The model under review builds one solid part; all positions refer to its coordinate system, in mm. A direction names the side the tool comes from. Coordinates: 2 decimals unless noted, no trailing zeros. Order: outer loops, then holes, each group sorted by start corner. A loop starts at its lowest first (then second) coordinate and runs counter-clockwise, first axis right, second up.
Autodesk Inventor part; units mm, degrees
ref_plane "YZ Plane" through (0, 0, 0) normal (1, 0, 0) x (0, 1, 0)
ref_plane "XZ Plane" through (0, 0, 0) normal (0, 1, 0) x (-1, 0, 0)
ref_plane "XY Plane" through (0, 0, 0) normal (0, 0, 1) x (1, 0, 0)
sketch "Sketch1" plane through (0, 0, 0) normal (0, 1, 0) x (-1, 0, 0)
  line L0 (0, 0) -> (-155, 0)
  line L1 (-155, 0) -> (-155, -65)
  line L2 (-155, -65) -> (0, -65)
  line L3 (0, -65) -> (0, 0)
  dimension "d0" = 155
  dimension "d1" = 65
extrude "Extrusion1" add sketch "Sketch1" along normal blind 4
sketch "Sketch2" plane through (0, 0, 0) normal (0, -1, 0) x (1, 0, 0)
  line L0 (155, 0) -> (155, -65)
  line L1 (0, 0) -> (155, 0)
  line L2 (0, -65) -> (0, 0)
  line L3 (155, -65) -> (0, -65)
  line L4 (3, -62) -> (3, -3)
  line L5 (3, -3) -> (152, -3)
  line L6 (152, -3) -> (152, -62)
  line L7 (152, -62) -> (3, -62)
  line L8 (152, -62) -> (143, -62)
  line L9 (143, -62) -> (143, -53)
  line L10 (143, -53) -> (152, -53)
  line L11 (152, -53) -> (152, -62)
  circle A0 centre (147.5, -57.5) radius 1.6
  dimension "d4" = 3
  dimension "d5" = 9
  dimension "d6" = 9
  dimension "d7" = 3.2
extrude "Extrusion2" cut sketch "Sketch2" against normal blind 4 contours A0
sketch "Sketch3" plane through (0, 4, 0) normal (0, 1, 0) x (1, 0, 0)
  circle A0 centre (147.5, 57.5) radius 1.6
  line L0 (155, 0) -> (155, 65)
  line L1 (155, 65) -> (0, 65)
  line L2 (0, 65) -> (0, 0)
  line L3 (0, 0) -> (155, 0)
  circle A1 centre (147.5, 57.5) radius 3
  dimension "d10" = 6
extrude "Extrusion3" cut sketch "Sketch3" against normal blind 1 contours A1
sketch "Sketch4" plane through (0, 0, 0) normal (0, -1, 0) x (1, 0, 0)
  circle A0 centre (147.5, -57.5) radius 1.6
  line L0 (155, 0) -> (155, -65)
  line L1 (0, 0) -> (155, 0)
  line L2 (0, -65) -> (0, 0)
  line L3 (155, -65) -> (0, -65)
  line L4 (3, -62) -> (3, -3)
  line L5 (3, -3) -> (152, -3)
  line L6 (152, -3) -> (152, -62)
  line L7 (152, -62) -> (3, -62)
  line L8 (152, -3) -> (143, -3)
  line L9 (143, -3) -> (143, -12)
  line L10 (143, -12) -> (152, -12)
  line L11 (152, -12) -> (152, -3)
  line L12 (3, -3) -> (12, -3)
  line L13 (12, -3) -> (12, -12)
  line L14 (12, -12) -> (3, -12)
  line L15 (3, -12) -> (3, -3)
  line L16 (3, -62) -> (12, -62)
  line L17 (12, -62) -> (12, -53)
  line L18 (12, -53) -> (3, -53)
  line L19 (3, -53) -> (3, -62)
  circle A1 centre (147.5, -7.5) radius 1.6
  circle A2 centre (7.5, -7.5) radius 1.6
  circle A3 centre (7.5, -57.5) radius 1.6
  dimension "d13" = 3
  dimension "d14" = 9
  dimension "d15" = 9
  dimension "d16" = 9
  dimension "d17" = 9
  dimension "d18" = 9
  dimension "d19" = 9
  dimension "d20" = 3.2
  dimension "d21" = 3.2
  dimension "d22" = 3.2
extrude "Extrusion4" cut sketch "Sketch4" against normal blind 4 contours A1 | A2 | A3
sketch "Sketch5" plane through (0, 4, 0) normal (0, 1, 0) x (1, 0, 0)
  circle A0 centre (7.5, 57.5) radius 1.6
  circle A1 centre (7.5, 7.5) radius 1.6
  circle A2 centre (147.5, 7.5) radius 1.6
  circle A3 centre (147.5, 57.5) radius 3
  line L0 (155, 0) -> (155, 65)
  line L1 (155, 65) -> (0, 65)
  line L2 (0, 65) -> (0, 0)
  line L3 (0, 0) -> (155, 0)
  circle A4 centre (7.5, 57.5) radius 3
  circle A5 centre (7.5, 7.5) radius 3
  circle A6 centre (147.5, 7.5) radius 3
  dimension "d25" = 6
  dimension "d26" = 6
  dimension "d27" = 6
extrude "Extrusion5" cut sketch "Sketch5" against normal blind 1 contours A4 | A5 | A6
fillet "Fillet1" radius 3 4 edges at (0, 2, 0) (0, 2, -65) (155, 2, 0) (155, 2, -65)
sketch "Sketch6" plane through (0, 4, 0) normal (0, 1, 0) x (1, 0, 0)
  line L0 (10, 25.325) -> (40, 25.325)
  line L1 (40, 25.325) -> (40, 39.675)
  line L2 (40, 39.675) -> (10, 39.675)
  line L3 (10, 39.675) -> (10, 25.325)
  line L4 (66.65, 25.325) -> (96.65, 25.325)
  line L5 (96.65, 25.325) -> (96.65, 39.675)
  line L6 (96.65, 39.675) -> (66.65, 39.675)
  line L7 (66.65, 39.675) -> (66.65, 25.325)
  point P0 (0, 0)
  dimension "d31" = 30
  dimension "d32" = 14.35
  dimension "d33" = 30
  dimension "d34" = 14.35
extrude "Extrusion6" cut sketch "Sketch6" against normal blind 4
fillet "Fillet2" radius 2 8 edges at (10, 2, -39.675) (40, 2, -39.675) (10, 2, -25.325) (40, 2, -25.325) (66.65, 2, -39.675) (96.65, 2, -39.675) (66.65, 2, -25.325) (96.65, 2, -25.325)
chamfer "Chamfer1" distance 0.3 angle 45 20 edges at (5.9, 0, -7.5) (10, 0, -32.5) (10.5858, 0, -25.9108) (25, 0, -25.325) (39.4142, 0, -25.9108) (40, 0, -32.5) (39.4142, 0, -39.0892) (25, 0, -39.675) (10.5858, 0, -39.0892) (67.2358, 0, -39.0892) (81.65, 0, -39.675) (96.0642, 0, -39.0892) (96.65, 0, -32.5) (96.0642, 0, -25.9108) (81.65, 0, -25.325) (67.2358, 0, -25.9108) (66.65, 0, -32.5) (5.9, 0, -57.5) (145.9, 0, -7.5) (145.9, 0, -57.5)
properties part number "arcade_box_lid_iteration3"
(1) Draft analysis for pull direction X (two halves, no side actions). For faces 4 (the face through (79, 2, -65)), 5 (the face through (25, 2, -25.325)), 6 (the face through (154.14, 2.03, -64.1)), 7 (the face through (66.65, 2, -33)), state which applies: released by +X, released by -X, zero draft, split by the parting line, or undercut.
A:
face 4: zero draft
face 5: undercut
face 6: released by +X
face 7: undercut
(2) We need section C-C, the plane z = -36. Write out the cut boundary in (x, y).
A:
outline: (0, 0) - (9.7, 0) - (10, 0.3) - (10, 4) - (0, 4) - close; (40, 0.3) - (40.3, 0) - (66.35, 0) - (66.65, 0.3) - (66.65, 4) - (40, 4) - close; (96.65, 0.3) - (96.95, 0) - (155, 0) - (155, 4) - (96.65, 4) - close
(3) Machinability: for faces 1 (the face through (40, 2, -32)), 2 (the face through (79, 4, -25)), 3 (the face through (10.27, 3.51, -6.35)), which of the approach directions +Z, -Z, +X, -X, +Y, -Y give a long, thin tool a straight path to every point of the face, cutting with its end or side? Answer none if there is none.
A:
face 1: +Y, -Y
face 2: +Z, -Z, +X, -X, +Y
face 3: +Y
(4) Wall thickness on probe 1 along X at (y, z) = (3.4, -7.5); probe 2 along X at (y, z) = (2.45, -7.5); probe 3 along Z at (x, y) = (7.5, 3.3): over which ranges is each line inside the solid? List them lowest first.
A:
probe 1: x = 0 to 4.5, 10.5 to 144.5, 150.5 to 155
probe 2: x = 0 to 5.9, 9.1 to 145.9, 149.1 to 155
probe 3: z = -65 to -60.5, -54.5 to -10.5, -4.5 to 0
(5) We need section A-A, the plane x = 147.5. Write out the cut boundary in (y, z), and give its area (3 significant figures).
A:
outline: (0, -65) - (4, -65) - (4, -60.5) - (3, -60.5) - (3, -59.1) - (0.3, -59.1) - (0, -59.4) - close; (0, -55.6) - (0.3, -55.9) - (3, -55.9) - (3, -54.5) - (4, -54.5) - (4, -10.5) - (3, -10.5) - (3, -9.1) - (0.3, -9.1) - (0, -9.4) - close; (0, -5.6) - (0.3, -5.9) - (3, -5.9) - (3, -4.5) - (4, -4.5) - (4, 0) - (0, 0) - close
area: 229 mm2
(6) For pin 1 Ø3.5 at (x, z) = (7.5, -57.5) entering from +Y, flat-tipped, find the tip position at first contact; note if it passes through.
A:
pin 1: stops at y = 3
(7) We need section D-D, the plane y = 2.3. Write out the cut boundary in (x, z) (3 decimals).
A:
outline: (0, -62) arc R3 ccw to (3, -65) - (152, -65) arc R3 ccw to (155, -62) - (155, -3) arc R3 ccw to (152, 0) - (3, 0) arc R3 ccw to (0, -3) - close; hole circle Ø3.2 at (7.5, -57.5); hole circle Ø3.2 at (7.5, -7.5); hole (10, -37.675) arc R2 ccw to (12, -39.675) - (38, -39.675) arc R2 ccw to (40, -37.675) - (40, -27.325) arc R2 ccw to (38, -25.325) - (12, -25.325) arc R2 ccw to (10, -27.325) - close; hole (66.65, -37.675) arc R2 ccw to (68.65, -39.675) - (94.65, -39.675) arc R2 ccw to (96.65, -37.675) - (96.65, -27.325) arc R2 ccw to (94.65, -25.325) - (68.65, -25.325) arc R2 ccw to (66.65, -27.325) - close; hole circle Ø3.2 at (147.5, -57.5); hole circle Ø3.2 at (147.5, -7.5)
(8) We need section B-B, the plane x = 83. Write out the cut boundary in (y, z) (3 decimals).
A:
outline: (0, -65) - (4, -65) - (4, -39.675) - (0.3, -39.675) - (0, -39.975) - close; (0, -25.025) - (0.3, -25.325) - (4, -25.325) - (4, 0) - (0, 0) - close
